Part print with two shaded views. Sizes in mm from the minimum x, y, z corner. A direction names the side the tool comes from. Round coordinates to 2 decimals unless told otherwise and drop trailing zeros. Loops run counter-clockwise (first coordinate to the right, second up) from the corner with the lowest first, then second, coordinate; pieces in that order, holes last. Notation, with made-up numbers: (51, 13.5) - (69, 13.5) arc R14 cw to (69, 28.5) - close; hole circle Ø2 at (-19.5, 75.25). An arc over 180 degrees is marked (long way). Write each question's results on one line, items separated by ' | '. Start each with the question number.
(1) Cut at B-B, the plane y = 10.75. List the corners of the cut face in (x, z), then the cut area to 3 significant figures.
(2) Tool access for the marked faces 4 and 5: list every direction of +Z, -Z, +X, -X, +Y, -Y with a clear straight run to the whole face (end or side of a thin tool).
(3) Cut at C-C, the plane x = 48. List the corners of the cut face in (y, z), then the cut area to 3 significant figures.
(4) Drill centre lines: L1, parallel to Y at x = 34, z = 2.45; L2, parallel to X at y = 4, z = 3.4; L3, parallel to X at y = 4.75, z = 3.2. Where is each one in solid material? Low to high.
(5) Cut at A-A, the plane z = 3.65. List the corners of the cut face in (x, y) (3 decimals), then the cut area to 3 significant figures.
(6) Flat gauge pins, fed straight in: P1, Ø3, axis at y = 6, z = 2.5, coming from the -X side (3 decimals); P2, Ø2.5, axis at x = 33, z = 3, coming from the +Y side; P3, Ø2, axis at x = 43, z = 0.5, coming from the +Y side. Where does each tip first touch, or does it go through?
(7) Cut at D-D, the plane x = 40.5. List the corners of the cut face in (y, z).
(8) Mould opens along X. For the marked faces 1, 2 and 3 say: released by +X, released by -X, zero draft, split by the parting line, or undercut.
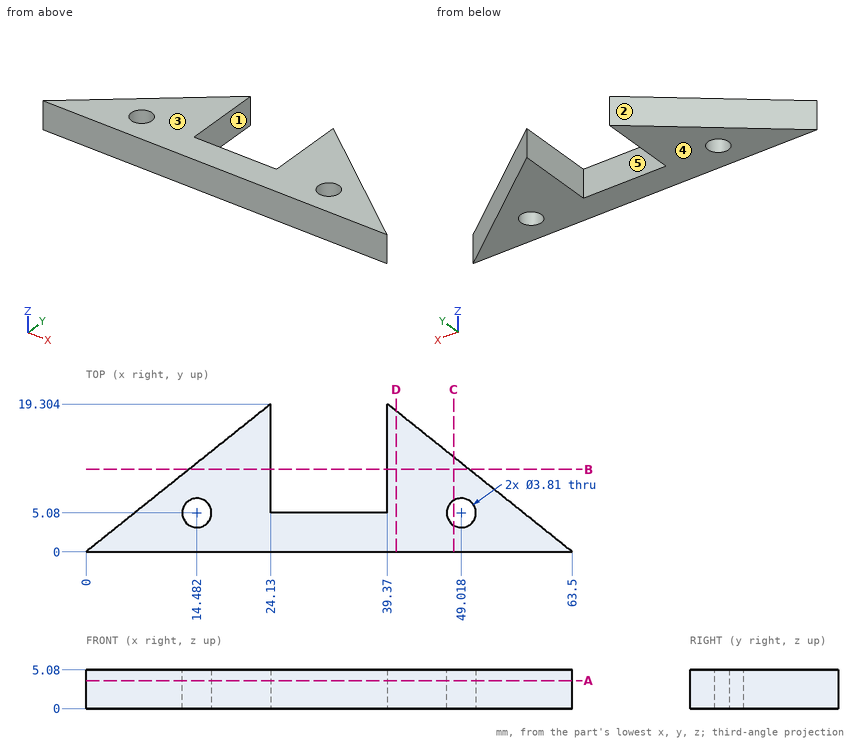
A:
1) outline: (13.44, 0) - (24.13, 0) - (24.13, 5.08) - (13.44, 5.08) - close; (39.37, 0) - (50.06, 0) - (50.06, 5.08) - (39.37, 5.08) - close | area: 109 mm2
2) face 4: -Z, +X, -X, +Y, -Y | face 5: +Z, -Z, +Y
3) outline: (0, 0) - (3.47, 0) - (3.47, 5.08) - (0, 5.08) - close; (6.69, 0) - (12.4, 0) - (12.4, 5.08) - (6.69, 5.08) - close | area: 46.6 mm2
4) L1: 0 to 5.08 | L2: 5 to 12.91, 16.05 to 47.45, 50.59 to 58.5 | L3: 5.94 to 12.61, 16.36 to 47.14, 50.89 to 57.56
5) outline: (0, 0) - (63.5, 0) - (39.37, 19.304) - (39.37, 5.08) - (24.13, 5.08) - (24.13, 19.304) - close; hole circle Ø3.81 at (14.482, 5.08); hole circle Ø3.81 at (49.018, 5.08) | area: 520 mm2
6) P1: x = 5.625 | P2: y = 5.08 | P3: y = 17.2
7) outline: (0, 0) - (18.4, 0) - (18.4, 5.08) - (0, 5.08) - close
8) face 1: undercut | face 2: released by -X | face 3: zero draft
